```python
from build123d import *

# Parameters (mm, degrees)
ESBO_O1_W                         = 40
ESBO_O1_H                         = 15
RESSALTO_EXTRUS_O1_DEPTH          = 3
ESBO_O3_W                         = 40
ESBO_O3_H                         = 15
RESSALTO_EXTRUS_O2_DEPTH          = 2
CORTE_EXTRUS_O1_REACH             = 26.418
CORTE_EXTRUS_O1_DIRECTION_2_REACH = 26.418
ESBO_O5_W                         = 20
ESBO_O5_H                         = 15
RESSALTO_EXTRUS_O4_DEPTH          = 60
CHANFRO1_SIZE                     = 19.068057482
CHANFRO1_SIZE_2                   = 16
FILETE4_R                         = 10
CORTE_EXTRUS_O2_DEPTH             = 81.237970309
FILETE5_R                         = 4.5


with BuildPart() as part:
    # Esboço1 → Ressalto-extrusão1 (new body)
    with BuildSketch(Plane.XY):
        with Locations((2.5, 1.5)):
            Rectangle(ESBO_O1_W, ESBO_O1_H)
    extrude(amount=-RESSALTO_EXTRUS_O1_DEPTH)

    # Esboço3 → Ressalto-extrusão2 (add)
    with BuildSketch(Plane.XY):
        with Locations((2.5, 1.5)):
            Rectangle(ESBO_O3_W, ESBO_O3_H)
    extrude(amount=RESSALTO_EXTRUS_O2_DEPTH)

    # Corte-extrusão1: up to this face of the body (flat: up to its plane)
    corte_extrus_o1_end = Plane(part.part.faces().sort_by_distance((2.5, 1.5, 2))[0])
    # Esboço2 → Corte-extrusão1 (cut, up to the picked face)
    with BuildSketch(Plane.XY, mode=Mode.PRIVATE) as corte_extrus_o1_sk1:
        with BuildLine():
            Line((0.085978459, 2.15), (-13, 2.15))
            Line((-13, 2.15), (-13, 0.85))
            Line((-13, 0.85), (0.085978459, 0.85))
            ThreePointArc((0.085978459, 0.85), (2.5, -1), (4.914021541, 0.85))
            Line((4.914021541, 0.85), (18, 0.85))
            Line((18, 0.85), (18, 2.15))
            Line((18, 2.15), (4.914021541, 2.15))
            ThreePointArc((4.914021541, 2.15), (2.5, 4), (0.085978459, 2.15))
        make_face()
    corte_extrus_o1_tool1 = split(extrude(corte_extrus_o1_sk1.sketch, amount=CORTE_EXTRUS_O1_REACH, mode=Mode.PRIVATE), bisect_by=corte_extrus_o1_end, keep=Keep.BOTH, mode=Mode.PRIVATE)
    add(corte_extrus_o1_tool1.solids().sort_by(Axis((2.5, 1.5, 0), (0, 0, 1)))[0], mode=Mode.SUBTRACT)

    # Corte-extrusão1 direction 2: up to this face of the body (flat: up to its plane)
    corte_extrus_o1_direction_2_end = Plane(part.part.faces().sort_by_distance((2.5, 1.5, -3))[0])
    # Esboço2 → Corte-extrusão1 direction 2 (cut, up to the picked face)
    with BuildSketch(Plane.XY, mode=Mode.PRIVATE) as corte_extrus_o1_direction_2_sk1:
        with BuildLine():
            Line((0.085978459, 2.15), (-13, 2.15))
            Line((-13, 2.15), (-13, 0.85))
            Line((-13, 0.85), (0.085978459, 0.85))
            ThreePointArc((0.085978459, 0.85), (2.5, -1), (4.914021541, 0.85))
            Line((4.914021541, 0.85), (18, 0.85))
            Line((18, 0.85), (18, 2.15))
            Line((18, 2.15), (4.914021541, 2.15))
            ThreePointArc((4.914021541, 2.15), (2.5, 4), (0.085978459, 2.15))
        make_face()
    corte_extrus_o1_direction_2_tool1 = split(extrude(corte_extrus_o1_direction_2_sk1.sketch, amount=-CORTE_EXTRUS_O1_DIRECTION_2_REACH, mode=Mode.PRIVATE), bisect_by=corte_extrus_o1_direction_2_end, keep=Keep.BOTH, mode=Mode.PRIVATE)
    add(corte_extrus_o1_direction_2_tool1.solids().sort_by(Axis((2.5, 1.5, 0), (0, 0, -1)))[0], mode=Mode.SUBTRACT)

    # Esboço5 → Ressalto-extrusão4 (add)
    with BuildSketch(Plane.ZY.offset(17.5)):
        with Locations((-0.5, 1.5)):
            Rectangle(ESBO_O5_W, ESBO_O5_H)
    extrude(amount=RESSALTO_EXTRUS_O4_DEPTH)

    # Chanfro1
    # the kernel refuses this chamfer: 19.068057482, 16 mm, written as the material it takes off along each edge
    with BuildSketch(Plane(origin=(-17.5, -55.146127732, 9.5), x_dir=(-0.9996889667359941, 0, 0.024939322090234247), z_dir=(0, 1, 0))) as chanfro1_piece_1_section:
        Polygon((CHANFRO1_SIZE * 0.99968896671, -CHANFRO1_SIZE * 0.0249393220896), (-CHANFRO1_SIZE_2 * 0.0249393220902, -CHANFRO1_SIZE_2 * 0.999688966736), (0, 0), align=None)
    chanfro1_piece_1 = extrude(amount=113.292255464, mode=Mode.PRIVATE)
    chanfro1_piece_1 = split(chanfro1_piece_1, bisect_by=Plane(origin=(-25.155035178, 1.5, 2), z_dir=(0, 0, 1)), keep=Keep.TOP, mode=Mode.PRIVATE)
    add(chanfro1_piece_1, mode=Mode.SUBTRACT)
    with BuildSketch(Plane(origin=(-17.5, -55.146127732, 9.5), x_dir=(-0.9996889667359941, 0, 0.024939322090234247), z_dir=(0, 1, 0))) as chanfro1_piece_2_section:
        Polygon((CHANFRO1_SIZE * 0.99968896671, -CHANFRO1_SIZE * 0.0249393220896), (-CHANFRO1_SIZE_2 * 0.0249393220902, -CHANFRO1_SIZE_2 * 0.999688966736), (0, 0), align=None)
    chanfro1_piece_2 = extrude(amount=113.292255464, mode=Mode.PRIVATE)
    chanfro1_piece_2 = split(chanfro1_piece_2, bisect_by=Plane(origin=(-18.373305927, 1.5, -3), z_dir=(0, 0, -1)), keep=Keep.TOP, mode=Mode.PRIVATE)
    add(chanfro1_piece_2, mode=Mode.SUBTRACT)
    with BuildSketch(Plane(origin=(-17.5, 58.146127732, -10.5), x_dir=(-0.9996889667359941, 0, -0.024939322090234247), z_dir=(0, -1, 0))) as chanfro1_piece_3_section:
        Polygon((CHANFRO1_SIZE * 0.99968896671, -CHANFRO1_SIZE * 0.0249393220896), (-CHANFRO1_SIZE_2 * 0.0249393220902, -CHANFRO1_SIZE_2 * 0.999688966736), (0, 0), align=None)
    chanfro1_piece_3 = extrude(amount=113.292255464, mode=Mode.PRIVATE)
    chanfro1_piece_3 = split(chanfro1_piece_3, bisect_by=Plane(origin=(-25.155035178, 1.5, -3), z_dir=(0, 0, -1)), keep=Keep.TOP, mode=Mode.PRIVATE)
    add(chanfro1_piece_3, mode=Mode.SUBTRACT)
    with BuildSketch(Plane(origin=(-17.5, 58.146127732, -10.5), x_dir=(-0.9996889667359941, 0, -0.024939322090234247), z_dir=(0, -1, 0))) as chanfro1_piece_4_section:
        Polygon((CHANFRO1_SIZE * 0.99968896671, -CHANFRO1_SIZE * 0.0249393220896), (-CHANFRO1_SIZE_2 * 0.0249393220902, -CHANFRO1_SIZE_2 * 0.999688966736), (0, 0), align=None)
    chanfro1_piece_4 = extrude(amount=113.292255464, mode=Mode.PRIVATE)
    chanfro1_piece_4 = split(chanfro1_piece_4, bisect_by=Plane(origin=(-18.373305927, 1.5, 2), z_dir=(0, 0, 1)), keep=Keep.TOP, mode=Mode.PRIVATE)
    add(chanfro1_piece_4, mode=Mode.SUBTRACT)

    # Filete4
    # the kernel refuses this fillet: 10 mm, written as the material it adds along each edge
    with BuildSketch(Plane(origin=(-27.629905537, -6, 2), x_dir=(1, 0, 0), z_dir=(0, 1, 0)), Plane(origin=(-27.629905537, 9, -3), x_dir=(1, 0, 0), z_dir=(0, -1, 0))) as filete4_piece_1:
        with BuildLine():
            CenterArc((FILETE4_R * 0.363970234266, -FILETE4_R), FILETE4_R, 90, 40)
            Line((-FILETE4_R * 0.27881737542, -FILETE4_R * 0.233955556881), (0, 0))
            Line((0, 0), (FILETE4_R * 0.363970234266, 0))
        make_face()
    extrude(amount=15)
    # the kernel refuses this fillet: 10 mm, written as the material it takes off along each edge
    with BuildSketch(Plane(origin=(-36.568057482, -15.099255857, 9.5), x_dir=(-1, 0, 0), z_dir=(0, 1, 0))) as filete4_2_piece_1:
        with BuildLine():
            CenterArc((FILETE4_R * 0.363970234266, -FILETE4_R), FILETE4_R, 90, 40)
            Line((-FILETE4_R * 0.27881737542, -FILETE4_R * 0.233955556881), (0, 0))
            Line((0, 0), (FILETE4_R * 0.363970234266, 0))
        make_face()
    extrude(amount=33.198511713, mode=Mode.SUBTRACT)
    with BuildSketch(Plane(origin=(-77.5, 9, 34.5), x_dir=(0, -1, 0), z_dir=(0, 0, -1))) as filete4_2_piece_2:
        with BuildLine():
            CenterArc((FILETE4_R, -FILETE4_R), FILETE4_R, 90, 90)
            Line((0, -FILETE4_R), (0, 0))
            Line((0, 0), (FILETE4_R, 0))
        make_face()
    extrude(amount=70, mode=Mode.SUBTRACT)
    with BuildSketch(Plane(origin=(-77.5, -6, -35.5), x_dir=(1, 0, 0), z_dir=(0, 0, 1))) as filete4_2_piece_3:
        with BuildLine():
            CenterArc((FILETE4_R, FILETE4_R), FILETE4_R, 180, 90)
            Line((0, FILETE4_R), (0, 0))
            Line((0, 0), (FILETE4_R, 0))
        make_face()
    extrude(amount=70, mode=Mode.SUBTRACT)
    with BuildSketch(Plane(origin=(-36.568057482, 18.099255857, -10.5), x_dir=(0.7660444431190706, 0, 0.6427876096864291), z_dir=(0, -1, 0))) as filete4_2_piece_4:
        with BuildLine():
            CenterArc((FILETE4_R * 0.363970234266, FILETE4_R), FILETE4_R, 230, 40)
            Line((-FILETE4_R * 0.27881737542, FILETE4_R * 0.233955556881), (0, 0))
            Line((0, 0), (FILETE4_R * 0.363970234266, 0))
        make_face()
    extrude(amount=33.198511713, mode=Mode.SUBTRACT)

    # Esboço6 → Corte-extrusão2 (cut, through all)
    with BuildSketch(Plane.XY.offset(9.5)):
        with BuildLine():
            Line((-43.207759824, 6), (-67.5, 6))
            ThreePointArc((-67.5, 6), (-71.468626967, 4.766281297), (-74.038348415, 1.5))
            ThreePointArc((-74.038348415, 1.5), (-71.468626967, -1.766281297), (-67.5, -3))
            Line((-67.5, -3), (-43.207759824, -3))
            Line((-43.207759824, -3), (-23.990203194, -3))
            Line((-23.990203194, -3), (-23.990203194, 6))
            Line((-23.990203194, 6), (-43.207759824, 6))
        make_face()
    extrude(amount=-CORTE_EXTRUS_O2_DEPTH, mode=Mode.SUBTRACT)

    # Filete5
    # the kernel refuses this fillet: 4.5 mm, written as the material it adds along each edge
    with BuildSketch(Plane(origin=(-23.990203194, 6, 13.25), x_dir=(0, -1, 0), z_dir=(0, 0, -1))) as filete5_piece_1_section:
        with BuildLine():
            CenterArc((FILETE5_R, FILETE5_R), FILETE5_R, 180, 90)
            Line((0, FILETE5_R), (0, 0))
            Line((0, 0), (FILETE5_R, 0))
        make_face()
    filete5_piece_1 = extrude(amount=27.5, mode=Mode.PRIVATE)
    filete5_piece_1 = filete5_piece_1 - Plane(origin=(-23.990203194, 5.729138272, 12), x_dir=(1, 0, 0), z_dir=(0, -1, 0)) * Cylinder(10, 73, mode=Mode.PRIVATE)
    filete5_piece_1 = filete5_piece_1 - Plane(origin=(-23.990203194, 5.729138272, -13), x_dir=(1, 0, 0), z_dir=(0, 1, 0)) * Cylinder(10, 73, mode=Mode.PRIVATE)
    add(filete5_piece_1)
    with BuildSketch(Plane(origin=(-23.990203194, -3, 13.25), x_dir=(-1, 0, 0), z_dir=(0, 0, -1))) as filete5_piece_2_section:
        with BuildLine():
            CenterArc((FILETE5_R, FILETE5_R), FILETE5_R, 180, 90)
            Line((0, FILETE5_R), (0, 0))
            Line((0, 0), (FILETE5_R, 0))
        make_face()
    filete5_piece_2 = extrude(amount=27.5, mode=Mode.PRIVATE)
    filete5_piece_2 = filete5_piece_2 - Plane(origin=(-23.990203194, -2.729138204, 12), x_dir=(1, 0, 0), z_dir=(0, -1, 0)) * Cylinder(10, 73, mode=Mode.PRIVATE)
    filete5_piece_2 = filete5_piece_2 - Plane(origin=(-23.990203194, -2.729138204, -13), x_dir=(1, 0, 0), z_dir=(0, 1, 0)) * Cylinder(10, 73, mode=Mode.PRIVATE)
    add(filete5_piece_2)
    # the kernel refuses this fillet: 4.5 mm, written as the material it takes off along each edge
    with BuildSketch(Plane(origin=(22.5, 9, -14.25), x_dir=(0, -1, 0), z_dir=(0, 0, 1))) as filete5_2_piece_1:
        with BuildLine():
            CenterArc((FILETE5_R, -FILETE5_R), FILETE5_R, 90, 90)
            Line((0, -FILETE5_R), (0, 0))
            Line((0, 0), (FILETE5_R, 0))
        make_face()
    extrude(amount=27.5, mode=Mode.SUBTRACT)
    with BuildSketch(Plane(origin=(22.5, -6, -14.25), x_dir=(0, 1, 0), z_dir=(0, 0, 1))) as filete5_2_piece_2:
        with BuildLine():
            CenterArc((FILETE5_R, FILETE5_R), FILETE5_R, 180, 90)
            Line((0, FILETE5_R), (0, 0))
            Line((0, 0), (FILETE5_R, 0))
        make_face()
    extrude(amount=27.5, mode=Mode.SUBTRACT)


solid = part.part
```
Input: part model. Units: mm. Frame: model coordinates. A direction names the side the tool comes from. Round coordinates to 2 decimals unless told otherwise and drop trailing zeros. Loops run counter-clockwise (first coordinate to the right, second up) from the corner with the lowest first, then second, coordinate; pieces in that order, holes last. Notation, with made-up numbers: (30.25, -16.75) -> (45.25, -16.75) arc R29 ccw to (45.25, 21.25) -> close; hole circle Ø5 at (3, -11.75). An arc over 180 degrees is marked (long way). Write each question's results on one line, items separated by ' | '.
1. Ray query, line 1 (Y direction, x = -62.5, z = -9); line 2 (X direction, y = 3, z = -1.5); line 3 (Z direction, x = 17, y = 7). Return the intervals inside material, ascending. Write a range as from..to.
Geometry results:
line 1: -6..-3, 6..9 | line 2: -76.67..-73.24, -24.25..0.5, 4.5..22.5 | line 3: -3..2
2. Section A-A (x = -50). Return loops of the section in (y, z).
Geometry results:
outline: (-6, -10.5) -> (-3, -10.5) -> (-3, 9.5) -> (-6, 9.5) -> close; (6, -10.5) -> (9, -10.5) -> (9, 9.5) -> (6, 9.5) -> close
3. Section C-C (x = 2.5). Return loops of the section in (y, z), and give its area (3 significant figures).
Geometry results:
outline: (-6, -3) -> (-1, -3) -> (-1, 2) -> (-6, 2) -> close; (4, -3) -> (9, -3) -> (9, 2) -> (4, 2) -> close | area: 50.0 mm2
4. Set-up query: faces 5 (the face through (-23.99, 1.6, -0.45)), 6 (the face through (-34, -6, -1)), 7 (the face through (0, 3, -3)). Return all of +Z, -Z, +X, -X, +Y, -Y with unobstructed straight access to the full face (end or side cutting, diameter ignored); none if empty.
Geometry results:
face 5: +Z, -Z | face 6: +Z, -Z, +X, -X, -Y | face 7: -Z, +X, +Y, -Y
5. First-contact query: P1, Ø1.5, axis at x = 9, y = 4.5, coming from the -Z side; P2, Ø4.5, axis at x = -4, y = -0.5, coming from the +Z side. Flat tips, straight axial feed; report the tip coordinate or a pass-through.
Geometry results:
P1: z = -3 | P2: z = 2
6. Section B-B (z = 0). Return loops of the section in (x, y), and give its area (3 significant figures).
Geometry results:
outline: (-77.18, 1.5) arc R10 ccw to (-67.5, -6) -> (18, -6) arc R4.5 ccw to (22.5, -1.5) -> (22.5, 4.5) arc R4.5 ccw to (18, 9) -> (-67.5, 9) arc R10 ccw to start; hole (-74.04, 1.5) arc R7 ccw to (-67.5, -3) -> (-28.49, -3) arc R4.5 ccw to (-28.49, 6) -> (-67.5, 6) arc R7 ccw to start; hole (-13, 0.85) -> (0.09, 0.85) arc R2.5 ccw to (4.91, 0.85) -> (18, 0.85) -> (18, 2.15) -> (4.91, 2.15) arc R2.5 ccw to (0.09, 2.15) -> (-13, 2.15) -> close | area: 970 mm2
7. Mould query, pull axis X, two halves, no side actions, for faces 1 (the face through (-58, -4, 9.5)), 2 (the face through (-48, -3, 0)), 3 (the face through (21.147, -4.717, -0.535)), 4 (the face through (11, 0.85, -1)). Classes: +X half, -X half, draft (parallel to the pull), parting line (faces both ways), or undercut.
Geometry results:
face 1: draft | face 2: undercut | face 3: +X half | face 4: undercut
